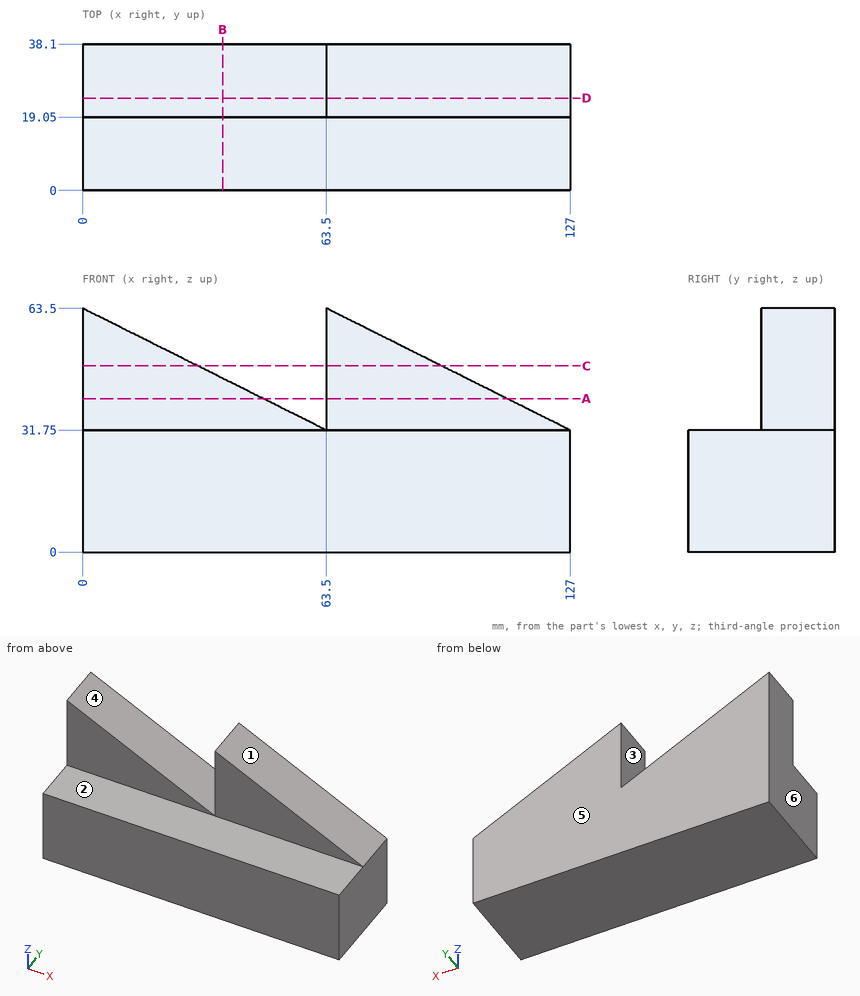
Geometry check sheet. Reference: drawing and pictorial views, mm from the part's lowest x, y, z. A direction names the side the tool comes from. Give positions to 0.01 mm unless a question says otherwise; leave off trailing zeros. Loops run counter-clockwise (first coordinate to the right, second up) from the corner with the lowest first, then second, coordinate; pieces in that order, holes last. Notation, with made-up numbers: M 55,39 L 74,39 A14 ccw 74,60 Z; hole C 81.5,-9 d5. An arc over 180 degrees is marked long. Use a Markdown table: item, result. Add a question column.
Q1. Sectioned sample at A-A, the plane z = 40. Record the cut outline in (x, y), then the cut area to 3 significant figures.
Q2. Sectioned sample at C-C, the plane z = 48.5. Record the cut outline in (x, y).
Q3. Scan lines: line 1 along Z through (x, y) = (11.5, 10.5); line 2 along X through (y, z) = (29.5, 32.5); line 3 along X through (y, z) = (23.5, 46.5). Record each from-to range of solid material in increasing order. Write a range as [from, to].
Q4. Mould release check, pull along X, two halves, no side actions. Record for the marked faces 4, 5 and 6: pulls with the +X half, pulls with the -X half, needs draft (parallel to the pull), parting line crosses it, or undercut.
Q5. Go/stop test with flat-tipped pins: pin 1 (5 mm diameter, centred on x = 51, y = 22.5, fed in from +Z); pin 2 (2 mm diameter, centred on x = 65, y = 29.5, fed in from +Z); pin 3 (15 mm diameter, centred on x = 68, y = 12.5, fed in from +Z). Record where each tip stops, or that it passes through.
Q6. Tool access check on the marked faces 1, 2 and 3. Record the directions out of +Z, -Z, +X, -X, +Y, -Y that give a thin tool (end or side, any length) a straight path to the whole face; none if there is none.
Q7. Sectioned sample at D-D, the plane y = 24. Record the cut outline in (x, z), then the cut area to 3 significant figures.
Q8. Sectioned sample at B-B, the plane x = 36.5. Record the cut outline in (y, z).
Verdict:
| question | item | result |
|---|---|---|
| 1 | outline | M 0,19.05 L 47,19.05 L 47,38.1 L 0,38.1 Z; M 63.5,19.05 L 110.5,19.05 L 110.5,38.1 L 63.5,38.1 Z |
| 1 | area | 1,790 mm^2 |
| 2 | outline | M 0,19.05 L 30,19.05 L 30,38.1 L 0,38.1 Z; M 63.5,19.05 L 93.5,19.05 L 93.5,38.1 L 63.5,38.1 Z |
| 3 | line 1 | [0, 31.75] |
| 3 | line 2 | [0, 62], [63.5, 125.5] |
| 3 | line 3 | [0, 34], [63.5, 97.5] |
| 4 | face 4 | undercut |
| 4 | face 5 | needs draft |
| 4 | face 6 | pulls with the -X half |
| 5 | pin 1 | z = 39.25 |
| 5 | pin 2 | z = 63.25 |
| 5 | pin 3 | z = 63.08 |
| 6 | face 1 | +Z, +X, +Y, -Y |
| 6 | face 2 | +Z, +X, -X, -Y |
| 6 | face 3 | +Z, +Y, -Y |
| 7 | outline | M 0,0 L 127,0 L 127,31.75 L 63.5,63.5 L 63.5,31.75 L 0,63.5 Z |
| 7 | area | 6,050 mm^2 |
| 8 | outline | M 0,0 L 38.1,0 L 38.1,45.25 L 19.05,45.25 L 19.05,31.75 L 0,31.75 Z |
